from build123d import *

# Parameters (mm, degrees)
BOSS_EXTRUDE1_DEPTH      = 20
BOSS_EXTRUDE1_DEPTH_BACK = 5
BOSS_EXTRUDE2_DEPTH      = 5
BOSS_EXTRUDE4_DEPTH      = 281


with BuildPart() as part:
    # Sketch1 → Boss-Extrude1 (new body, two sides)
    with BuildSketch(Plane.XY) as boss_extrude1_sk:
        with BuildLine():
            Line((0, 25), (0, 17))
            ThreePointArc((0, 17), (-17, 0), (0, -17))
            Line((0, -17), (0, -25))
            ThreePointArc((0, -25), (-25, 0), (0, 25))
        make_face()
    extrude(amount=BOSS_EXTRUDE1_DEPTH)
    extrude(boss_extrude1_sk.sketch, amount=-BOSS_EXTRUDE1_DEPTH_BACK)

    # Sketch2 → Boss-Extrude2 (add)
    with BuildSketch(Plane.XY):
        with BuildLine():
            Line((0, 25), (0, 77))
            Line((0, 77), (-65, 77))
            Line((-65, 77), (-65, 32.113081447))
            ThreePointArc((-65, 32.113081447), (-61.581037686, -38.262590053), (0, -72.5))
            Line((0, -72.5), (0, -25))
            ThreePointArc((0, -25), (-25, 0), (0, 25))
        make_face()
    extrude(amount=BOSS_EXTRUDE2_DEPTH)


with BuildPart() as body_2:
    # Mirror2: mirrored copy
    add(part.part.mirror(Plane.XY.offset(-140.5)))


with BuildPart() as part_1:
    add(part.part)

    add(body_2.part)  # Boss-Extrude4 merges body 2
    # Sketch3 → Boss-Extrude4 (add)
    with BuildSketch(Plane(origin=(0, 0, 0), x_dir=(-1, 0, 0), z_dir=(0, 0, -1))):
        with BuildLine():
            Line((60, 77), (60, 30.923292192))
            ThreePointArc((60, 30.923292192), (57.634938288, -35.134938288), (0, -67.5))
            Line((0, -67.5), (0, -72.5))
            ThreePointArc((0, -72.5), (61.581037686, -38.262590053), (65, 32.113081447))
            Line((65, 32.113081447), (65, 77))
            Line((65, 77), (60, 77))
        make_face()
    extrude(amount=BOSS_EXTRUDE4_DEPTH)


solid = part_1.part
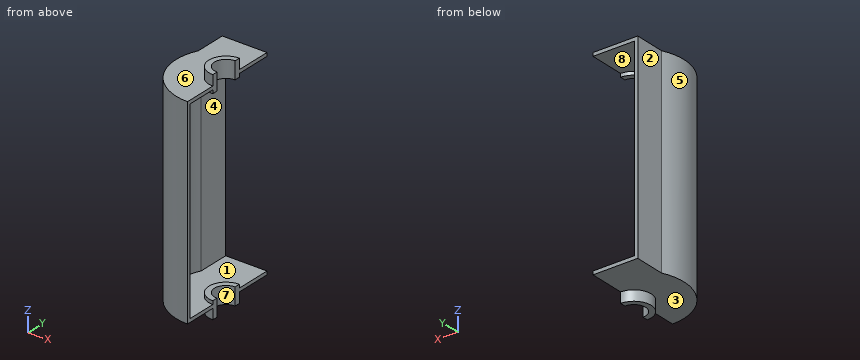
Verification items for the finished model (mm, model axes). Face numbers are marked on the shaded views. A direction names the side the tool comes from. Coordinates: 2 decimals unless noted, no trailing zeros. Order: outer loops, then holes, each group sorted by start corner. A loop starts at its lowest first (then second) coordinate and runs counter-clockwise, first axis right, second up.
Item 1: Section check A-A, the plane y = 0. Enter the section's corners in (x, z), then the cut area to 3 significant figures.
Filled in:
outline: (-72.5, -286) - (-25, -286) - (-25, -301) - (-17, -301) - (-17, -276) - (-25, -276) - (-25, -281) - (-67.5, -281) - (-67.5, 0) - (-25, 0) - (-25, -5) - (-17, -5) - (-17, 20) - (-25, 20) - (-25, 5) - (-72.5, 5) - close
area: 2,280 mm2
Item 2: Section check B-B, the plane x = -35. Enter the section's corners in (y, z), then the cut area to 3 significant figures.
Filled in:
outline: (-63.49, -286) - (77, -286) - (77, -281) - (-57.72, -281) - (-57.72, 0) - (77, 0) - (77, 5) - (-63.49, 5) - close
area: 3,030 mm2
Item 3: Section check C-C, the plane z = -17. Enter the section's corners in (x, y), then the cut area to 3 significant figures.
Filled in:
outline: (-65, 32.11) arc R72.5 ccw to (0, -72.5) - (0, -67.5) arc R67.5 cw to (-60, 30.92) - (-60, 77) - (-65, 77) - close
area: 941 mm2
Item 4: Release check for a two-part mould opening along Z. For the marked faces 6, 7 and 8 record: +Z half, -Z half, draft (parallel to the pull), parting line (faces both ways), or undercut.
Filled in:
face 6: +Z half
face 7: draft
face 8: undercut
Item 5: Depth check by flat-ended pin: pin 1 (12 mm diameter, centred on x = -38, y = -32, fed in from -Z); pin 2 (22.5 mm diameter, centred on y = 50.5, z = -157, fed in from -X); pin 3 (1.5 mm diameter, centred on x = -21, y = 45.5, fed in from +Z). Enter the tip coordinate at first touch or a pass-through.
Filled in:
pin 1: stops at z = -286
pin 2: stops at x = -65
pin 3: stops at z = 5
Item 6: Access from +Z, -Z, +X, -X, +Y, -Y to the whole of each face (thin tool, end or side, straight path). Record for the marked faces 1, 2, 3, 4 and 5.
Filled in:
face 1: none
face 2: +Z, -Z, -X, +Y
face 3: -Z, -X
face 4: +X, +Y
face 5: +Z, -Z, -X
Item 7: Material ranges on L1, parallel to Z at x = -51.5, y = -8.5; L2, parallel to Z at x = -11, y = 19.5; L3, parallel to Z at x = -64.5, y = 58, recorded low to high.
Filled in:
L1: z = -286 to -281, 0 to 5
L2: z = -301 to -276, -5 to 20
L3: z = -286 to 5
Item 8: Section check D-D, the plane y = 67. Enter the section's corners in (x, z).
Filled in:
outline: (-65, -286) - (0, -286) - (0, -281) - (-60, -281) - (-60, 0) - (0, 0) - (0, 5) - (-65, 5) - close
